Geometry check sheet. Reference: the model listing, model coordinates, mm. A direction names the side the tool comes from. Coordinates: 2 decimals unless noted, no trailing zeros. Loops run counter-clockwise (first coordinate to the right, second up) from the corner with the lowest first, then second, coordinate; pieces in that order, holes last.
Autodesk Inventor part; units mm, degrees
ref_plane "YZ Plane" through (0, 0, 0) normal (1, 0, 0) x (0, 1, 0)
ref_plane "XZ Plane" through (0, 0, 0) normal (0, 1, 0) x (-1, 0, 0)
ref_plane "XY Plane" through (0, 0, 0) normal (0, 0, 1) x (1, 0, 0)
sketch "Sketch1" plane through (0, 0, 0) normal (0, 1, 0) x (-1, 0, 0)
  circle A0 centre (0, 0) radius 25
  dimension "d0" = 50
extrude "Extrusion1" add sketch "Sketch1" along normal blind 5
chamfer "Chamfer1" distance 4 angle 45 1 edges at (25, 5, 0)
sketch "Sketch2" plane through (0, 5, 0) normal (0, 1, 0) x (1, 0, 0)
  circle A0 centre (0, 0) radius 2
  circle A1 centre (0, 0) radius 4.5
  dimension "d6" = 4
  dimension "d7" = 9
extrude "Extrusion2" add sketch "Sketch2" along normal blind 10
chamfer "Chamfer2" distance 2 angle 45 1 edges at (-4.5, 5, 0)
chamfer "Chamfer3" distance 2 angle 45 1 edges at (-2, 15, 0)
sketch "Sketch3" plane through (0, 5, 0) normal (0, 1, 0) x (1, 0, 0)
  line L0 (17, 2.5) -> (20, 2.5)
  line L1 (20, 2.5) -> (20, -2.5)
  line L2 (20, -2.5) -> (17, -2.5)
  line L3 (17, -2.5) -> (17, 2.5)
  point P0 (0, 0)
  dimension "d16" = 3
  dimension "d17" = 5
  dimension "d29" = 17
extrude "Extrusion3" add sketch "Sketch3" along normal blind 40
sketch "Sketch4" plane through (17, 5, -2.5) normal (-1, 0, 0) x (0, 0, 1)
  line L0 (5, 40) -> (0, 40)
  line L1 (5, 0) -> (5, 40)
  line L2 (0, 40) -> (5, 40)
  line L3 (5, 40) -> (5, 37)
  line L4 (5, 37) -> (0, 37)
  line L5 (0, 37) -> (0, 40)
  point P0 (2.5, -5)
  dimension "d20" = 3
extrude "Extrusion4" add sketch "Sketch4" along normal blind 3
chamfer "Chamfer4" distance 2 angle 45 1 edges at (14, 45, 0)
mirror "Mirror1" about plane through (0, 0, 0) normal (1, 0, 0) of "Extrusion3", "Chamfer4", "Extrusion4"
chamfer "Chamfer6" distance 0.5 angle 45 8 edges at (20, 5, 0) (18.5, 5, 2.5) (18.5, 5, -2.5) (17, 5, 0) (-17, 5, 0) (-18.5, 5, 2.5) (-20, 5, 0) (-17, 23.5, -2.5)
properties part number "supportPoint2"
1) Material ranges on probe 1 along X at (y, z) = (11, 0); probe 2 along Z at (x, y) = (0, 8.5); probe 3 along Y at (x, z) = (-13, 15.5), recorded low to high.
Data:
probe 1: x = -20 to -17, -4.5 to -2, 2 to 4.5, 17 to 20
probe 2: z = -4.5 to -2, 2 to 4.5
probe 3: y = 0 to 5
2) Section check B-B on x = 0. Record the cut outline in (y, z).
Data:
outline: (0, -25) - (1, -25) - (5, -21) - (5, -6.5) - (7, -4.5) - (15, -4.5) - (15, -4) - (13, -2) - (5, -2) - (5, 2) - (13, 2) - (15, 4) - (15, 4.5) - (7, 4.5) - (5, 6.5) - (5, 21) - (1, 25) - (0, 25) - close
3) Section check A-A on y = 18. Record the cut outline in (x, z).
Data:
outline: (-20, -2.5) - (-17.5, -2.5) - (-17, -2) - (-17, 2.5) - (-20, 2.5) - close; (17, -2.5) - (20, -2.5) - (20, 2.5) - (17, 2.5) - close
4) Mould release check, pull along Y, two halves, no side actions. Record for faces 1 (the flat face through (-18, 45, 0)), 2 (the flat face through (-18, 30, -2.5)), 3 (the flat face through (-17, 23, 0)): +Y half, -Y half, draft (parallel to the pull), parting line (faces both ways), or undercut.
Data:
face 1: +Y half
face 2: draft
face 3: undercut
5) Depth check by flat-ended pin: pin 1 (8 mm diameter, centred on y = 37, z = -5.5, fed in from -X); pin 2 (1.3 mm diameter, centred on y = 18.5, z = 0.5, fed in from +X); pin 3 (1 mm diameter, centred on x = 13, z = 3.5, fed in from +Y); pin 4 (3 mm diameter, centred on y = 19.5, z = -4.5, fed in from +X). Enter the tip coordinate at first touch or a pass-through.
Data:
pin 1: stops at x = -20
pin 2: stops at x = 20
pin 3: stops at y = 5
pin 4: passes through
6) Access from +Z, -Z, +X, -X, +Y, -Y to the whole of each face (thin tool, end or side, straight path). Record for faces 4 (the cylindrical face through (0, 9, -2)), 5 (the flat face through (-3, 15, 3)), 6 (the flat face through (17, 23, 0)).
Data:
face 4: +Y
face 5: +Z, -Z, +Y
face 6: +Z, -Z
